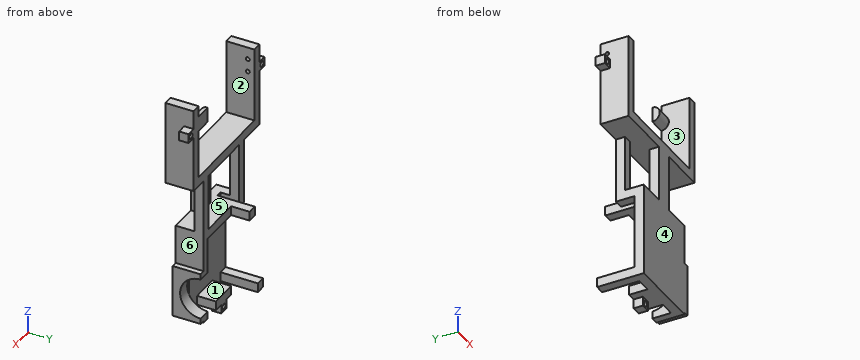
```python
from build123d import *

# Parameters (mm, degrees)
SKETCH1_W            = 40
SKETCH1_H            = 50
BOSS_EXTRUDE1_DEPTH  = 5
SKETCH4_W            = 5
SKETCH4_H            = 5
BOSS_EXTRUDE4_DEPTH  = 20
SKETCH4_4_W          = 15
SKETCH4_4_H          = 5
SKETCH4_4_W_2        = 5
BOSS_EXTRUDE5_DEPTH  = 10
CUT_EXTRUDE2_DEPTH   = 4
BOSS_EXTRUDE7_START  = 3
BOSS_EXTRUDE7_DEPTH  = 3
SKETCH10_W           = 5
SKETCH10_H           = 5
BOSS_EXTRUDE9_DEPTH  = 5
SKETCH11_R           = 1.5
CUT_EXTRUDE3_DEPTH   = 5
SKETCH12_W           = 5
SKETCH12_H           = 5
SKETCH12_W_2         = 10
BOSS_EXTRUDE10_DEPTH = 30
SKETCH13_W           = 40
SKETCH13_H           = 15
BOSS_EXTRUDE11_DEPTH = 5
SKETCH14_W           = 5
SKETCH14_H           = 15
BOSS_EXTRUDE12_DEPTH = 10
SKETCH15_W           = 5
SKETCH15_H           = 15
BOSS_EXTRUDE13_DEPTH = 15
SKETCH16_W           = 5
SKETCH16_H           = 15
BOSS_EXTRUDE14_DEPTH = 40
BOSS_EXTRUDE15_DEPTH = 9
SKETCH18_W           = 5
SKETCH18_H           = 5
BOSS_EXTRUDE16_DEPTH = 5
SKETCH19_R           = 1.5
CUT_EXTRUDE4_DEPTH   = 5
SKETCH20_W           = 5
SKETCH20_H           = 5
BOSS_EXTRUDE17_DEPTH = 5
SKETCH21_R           = 1.5
CUT_EXTRUDE5_DEPTH   = 5
SKETCH24_R           = 1.05
CUT_EXTRUDE6_DEPTH   = 5


with BuildPart() as part:
    # Sketch1 → Boss-Extrude1 (new body)
    with BuildSketch(Plane(origin=(0, 0, 0), x_dir=(1, 0, 0), z_dir=(0, 1, 0))):
        Rectangle(SKETCH1_W, SKETCH1_H)
    extrude(amount=BOSS_EXTRUDE1_DEPTH)

    # Sketch4 → Boss-Extrude4 (add)
    with BuildSketch(Plane(origin=(0, 5, 0), x_dir=(1, 0, 0), z_dir=(0, 1, 0))):
        with Locations((-9.5, -22.5)):
            Rectangle(SKETCH4_W, SKETCH4_H)
        with Locations((-17.5, 22.5)):
            Rectangle(SKETCH4_W, SKETCH4_H)
    extrude(amount=BOSS_EXTRUDE4_DEPTH)

    # Sketch4_4 → Boss-Extrude5 (add)
    with BuildSketch(Plane(origin=(0, 5, 0), x_dir=(1, 0, 0), z_dir=(0, 1, 0))):
        Polygon((20, -25), (20, 25), (16, 25), (16, -20), (-7, -20), (-7, -25), align=None)
        with Locations((0.5, 22.5)):
            Rectangle(SKETCH4_4_W, SKETCH4_4_H)
        with Locations((-17.5, -22.5)):
            Rectangle(SKETCH4_4_W_2, SKETCH4_4_H)
    extrude(amount=BOSS_EXTRUDE5_DEPTH)

    # Sketch7 → Cut-Extrude2 (cut)
    with BuildSketch(Plane(origin=(20, 0, 0), x_dir=(0, 0, -1), z_dir=(1, 0, 0))):
        with BuildLine():
            Line((-1, 15), (21, 15))
            ThreePointArc((21, 15), (10, 4), (-1, 15))
        make_face()
    extrude(amount=-CUT_EXTRUDE2_DEPTH, mode=Mode.SUBTRACT)

    # Sketch8 → Boss-Extrude7 (add)
    with BuildSketch(Plane(origin=(20, 0, 0), x_dir=(0, 0, -1), z_dir=(1, 0, 0)).offset(BOSS_EXTRUDE7_START)):
        with BuildLine():
            Line((-1, 15), (-4, 15))
            Line((-4, 15), (-4, 0))
            Line((-4, 0), (24, 0))
            Line((24, 0), (24, 15))
            Line((24, 15), (21, 15))
            ThreePointArc((21, 15), (10, 4), (-1, 15))
        make_face()
    extrude(amount=-BOSS_EXTRUDE7_DEPTH)

    # Sketch10 → Boss-Extrude9 (add)
    with BuildSketch(Plane(origin=(0, 0, -25), x_dir=(-1, 0, 0), z_dir=(0, 0, -1))):
        with Locations((0, 12.5)):
            Rectangle(SKETCH10_W, SKETCH10_H)
    extrude(amount=BOSS_EXTRUDE9_DEPTH)

    # Sketch11 → Cut-Extrude3 (cut)
    with BuildSketch(Plane.XZ.offset(-10)):
        with Locations(Location((0, -27.5, 0), (0, 0, 270))):
            Circle(SKETCH11_R)
    extrude(amount=-CUT_EXTRUDE3_DEPTH, mode=Mode.SUBTRACT)

    # Sketch12 → Boss-Extrude10 (add)
    with BuildSketch(Plane.XY.offset(25)):
        with Locations((-17.5, 12.5)):
            Rectangle(SKETCH12_W, SKETCH12_H)
        with Locations((17.5, 12.5)):
            Rectangle(SKETCH12_W, SKETCH12_H)
        with Locations((0, 2.5)):
            Rectangle(SKETCH12_W_2, SKETCH12_H)
    extrude(amount=BOSS_EXTRUDE10_DEPTH)

    # Sketch13 → Boss-Extrude11 (add)
    with BuildSketch(Plane.XY.offset(55)):
        with Locations((0, 7.5)):
            Rectangle(SKETCH13_W, SKETCH13_H)
    extrude(amount=BOSS_EXTRUDE11_DEPTH)

    # Sketch14 → Boss-Extrude12 (add)
    with BuildSketch(Plane(origin=(20, 0, 0), x_dir=(0, 0, -1), z_dir=(1, 0, 0))):
        with Locations((-57.5, 7.5)):
            Rectangle(SKETCH14_W, SKETCH14_H)
    extrude(amount=BOSS_EXTRUDE12_DEPTH)

    # Sketch15 → Boss-Extrude13 (add)
    with BuildSketch(Plane.ZY.offset(20)):
        with Locations((57.5, 7.5)):
            Rectangle(SKETCH15_W, SKETCH15_H)
    extrude(amount=BOSS_EXTRUDE13_DEPTH)

    # Sketch16 → Boss-Extrude14 (add)
    with BuildSketch(Plane.XY.offset(60)):
        with Locations((-32.5, 7.5)):
            Rectangle(SKETCH16_W, SKETCH16_H)
        with Locations((27.5, 7.5)):
            Rectangle(SKETCH16_W, SKETCH16_H)
    extrude(amount=BOSS_EXTRUDE14_DEPTH)

    # Sketch17 → Boss-Extrude15 (add)
    with BuildSketch(Plane.ZY.offset(-25)):
        with BuildLine():
            Line((86, 15), (94, 15))
            ThreePointArc((94, 15), (90, 11), (86, 15))
        make_face()
    extrude(amount=BOSS_EXTRUDE15_DEPTH)

    # Sketch18 → Boss-Extrude16 (add)
    with BuildSketch(Plane.ZY.offset(35)):
        with Locations((87.5, 12.5)):
            Rectangle(SKETCH18_W, SKETCH18_H)
    extrude(amount=BOSS_EXTRUDE16_DEPTH)

    # Sketch19 → Cut-Extrude4 (cut)
    with BuildSketch(Plane.XZ.offset(-10)):
        with Locations(Location((-37.5, 87.5, 0), (0, 0, 270))):
            Circle(SKETCH19_R)
    extrude(amount=-CUT_EXTRUDE4_DEPTH, mode=Mode.SUBTRACT)

    # Sketch20 → Boss-Extrude17 (add)
    with BuildSketch(Plane(origin=(30, 0, 0), x_dir=(0, 0, -1), z_dir=(1, 0, 0))):
        with Locations((-87.5, 12.5)):
            Rectangle(SKETCH20_W, SKETCH20_H)
    extrude(amount=BOSS_EXTRUDE17_DEPTH)

    # Sketch21 → Cut-Extrude5 (cut)
    with BuildSketch(Plane.XZ.offset(-10)):
        with Locations(Location((32.5, 87.5, 0), (0, 0, 270))):
            Circle(SKETCH21_R)
    extrude(amount=-CUT_EXTRUDE5_DEPTH, mode=Mode.SUBTRACT)

    # Sketch24 → Cut-Extrude6 (cut)
    with BuildSketch(Plane(origin=(-30, 0, 0), x_dir=(0, 0, -1), z_dir=(1, 0, 0))):
        with Locations(Location((-93.5, 11.5, 0), (0, 0, 90))):
            Circle(SKETCH24_R)
        with Locations(Location((-86.5, 11.5, 0), (0, 0, 90))):
            Circle(SKETCH24_R)
    extrude(amount=-CUT_EXTRUDE6_DEPTH, mode=Mode.SUBTRACT)


solid = part.part
```
The listing builds one solid part. Answer for the finished solid, in the listing's coordinates (mm). Face numbers are marked on the shaded views. A direction names the side the tool comes from. Give positions to 0.01 mm unless a question says otherwise; leave off trailing zeros. Order: outer loops, then holes, each group sorted by start corner. A loop starts at its lowest first (then second) coordinate and runs counter-clockwise, first axis right, second up. Notation, with made-up numbers: (-12.75, -35.75) -> (22.25, -35.75) arc R26 ccw to (22.25, 3.25) -> close; hole circle Ø1 at (4.25, 80.5). An arc over 180 degrees is marked (long way). One line per item, written item: value.
1) A tool of negligible diameter and unlimited length cuts with its end or side. For the marked faces 1, 2 and 3, from which of +Z, -Z, +X, -X, +Y, -Y can it reach the whole face along a straight path? Write none if from no direction.
Reported:
face 1: -X, +Y
face 2: +Z, +Y, -Y
face 3: -Y
2) Find the intervals of material crossed by line 1 (X direction, y = 11.55, z = 87.5); line 2 (Z direction, x = -31.3, y = 11.5); line 3 (X direction, y = 11.05, z = 87.5), in increasing order.
Reported:
line 1: x = -40 to -39, -36 to -35, 25 to 31, 34 to 35
line 2: z = 55 to 85.45, 87.55 to 92.45, 94.55 to 100
line 3: x = -40 to -39, -36 to -30, 25 to 31, 34 to 35
3) Determine the mould class of the marked faces 4, 5 and 6 for opening direction X: pulls with the +X half, pulls with the -X half, needs draft (parallel to the pull), parting line crosses it, or undercut.
Reported:
face 4: needs draft
face 5: undercut
face 6: pulls with the +X half
4) Find section B-B, the plane x = -37.5. Determine the outline of the cut face in (y, z), plus the area to 3 significant figures.
Reported:
outline: (10, 85) -> (15, 85) -> (15, 86) -> (10, 86) -> close; (10, 89) -> (15, 89) -> (15, 90) -> (10, 90) -> close
area: 10.0 mm^2
5) Find section C-C, the plane z = 16.5. Determine the outline of the cut face in (x, y), plus the area to 3 significant figures.
Reported:
outline: (-20, 0) -> (20, 0) -> (20, 15) -> (16, 15) -> (16, 5) -> (-20, 5) -> close
area: 240 mm^2
6) Flat-ended cylindrical pins translate along their axes: P1, Ø5, axis at y = 11, z = 12.5, coming from the +X side; P2, Ø2.5, axis at x = -17, z = 42, coming from the -Y side; P3, Ø1, axis at y = 11, z = 42, coming from the -X side. Find the tip coordinate at first contact, or state that the pin passes through.
Reported:
P1: stops at x = 20
P2: stops at y = 10
P3: stops at x = -20
7) Find section D-D, the plane x = 28.5. Determine the outline of the cut face in (y, z).
Reported:
outline: (0, 55) -> (15, 55) -> (15, 100) -> (0, 100) -> close
8) Find section A-A, the plane z = -27.5. Determine the outline of the cut face in (x, y).
Reported:
outline: (-2.5, 10) -> (-1.5, 10) -> (-1.5, 15) -> (-2.5, 15) -> close; (1.5, 10) -> (2.5, 10) -> (2.5, 15) -> (1.5, 15) -> close
